Read the model definition and answer for the solid it produces. Units are mm, in the model's axes. A direction names the side the tool comes from. Coordinates: 2 decimals unless noted, no trailing zeros. Loops run counter-clockwise (first coordinate to the right, second up) from the corner with the lowest first, then second, coordinate; pieces in that order, holes last. Notation, with made-up numbers: (-6.75, 63) -> (11.25, 63) arc R13 ccw to (11.25, 69) -> close; hole circle Ø6 at (-26, -1.75). An arc over 180 degrees is marked (long way). Answer in a Markdown table with one row per item.
```python
from build123d import *

# Parameters (mm, degrees)
BASE_EXTRUSION_DEPTH    = 5.04
ESQUISSE3_R             = 2.5
ENL_V_MAT_EXTRU_1_DEPTH = 8.920538702
ESQUISSE5_R             = 2.5
ESQUISSE5_R_2           = 2
BOSS_EXTRU_1_DEPTH      = 5.04


with BuildPart() as part:
    # Esquisse1 → Base-Extrusion (new body)
    with BuildSketch(Plane.XY):
        Polygon((4, -2.309401077), (4, 2.309401077), (0, 4.618802154), (-4, 2.309401077), (-4, -2.309401077), (0, -4.618802154), align=None)
    extrude(amount=-BASE_EXTRUSION_DEPTH)

    # Esquisse2 → Enlèvement de matière-Révolution1 (revolve, cut)
    with BuildSketch(Plane(origin=(0, 0, 0), x_dir=(1, 0, 0), z_dir=(0, 1, 0))):
        Polygon((-4, 0), (-9.364768035, 0), (-9.364768035, 5.04), (-4, 5.04), (-8.364768035, 2.52), align=None)
    revolve(axis=Axis((0, 0, -5.04), (0, 0, 1)), mode=Mode.SUBTRACT)

    # Esquisse3 → Enlèv. mat.-Extru.1 (cut, through all)
    with BuildSketch(Plane.XY):
        Circle(ESQUISSE3_R)
    extrude(amount=-ENL_V_MAT_EXTRU_1_DEPTH, mode=Mode.SUBTRACT)

    # Esquisse4 → Boss.-Révol.1 (revolve)
    with BuildSketch(Plane(origin=(0, 0, 0), x_dir=(0, 0, -1), z_dir=(1, 0, 0)), mode=Mode.PRIVATE) as boss_r_vol_1_sk:
        with BuildLine():
            Line((5.04, 4), (5.67, 4))
            ThreePointArc((5.67, 4), (6.115477272, 3.815477272), (6.3, 3.37))
            Line((6.3, 3.37), (6.3, 3.154700538))
            Line((6.3, 3.154700538), (5.775, 3.154700538))
            Line((5.775, 3.154700538), (5.775, 2.309401077))
            Line((5.775, 2.309401077), (5.04, 2.309401077))
            Line((5.04, 2.309401077), (5.04, 4))
        make_face()
    revolve(boss_r_vol_1_sk.sketch.rotate(Axis((0, 0, 0), (0, 0, -1)), 90), axis=Axis((0, 0, 0), (0, 0, -1)))

    # Esquisse5 → Boss.-Extru.1 (add)
    with BuildSketch(Plane.XY):
        Circle(ESQUISSE5_R)
        Circle(ESQUISSE5_R_2, mode=Mode.SUBTRACT)
    extrude(amount=-BOSS_EXTRU_1_DEPTH)


solid = part.part
```
1. A cutting plane is placed at A-A on z = -1.5. Give the vertices of the cut face in (x, y).
A:
| item | result |
|---|---|
| outline | (-4, -2.31) -> (0, -4.62) -> (4, -2.31) -> (4, 2.31) -> (0, 4.62) -> (-4, 2.31) -> close; hole circle Ø4 at (0, 0) |
2. The mould has two halves that part along Y. Classify faces 1 (the cylindrical face through (-0.867, 3.905, -5.359)), 2 (the cylindrical face through (0, -2, -2)), 3 (the conical face through (3.6, 2.07, -4.95)), 4 (the cylindrical face through (1.456, 2.799, -6.034)): pulls with the +Y half, pulls with the -Y half, needs draft (parallel to the pull), parting line crosses it, or undercut.
A:
| item | result |
|---|---|
| face 1 | parting line crosses it |
| face 2 | undercut |
| face 3 | pulls with the +Y half |
| face 4 | undercut |
3. A cutting plane is placed at B-B on z = -5.5. Give the vertices of the cut face in (x, y).
A:
| item | result |
|---|---|
| outline | circle Ø8 at (0, 0); hole circle Ø4.62 at (0, 0) |
4. A tool of negligible diameter and unlimited length cuts with its end or side. For faces 5 (the cylindrical face through (1.066, 2.049, -5.402)), 6 (the flat face through (2.028, 3.448, -2.485)), from which of +Z, -Z, +X, -X, +Y, -Y can it reach the whole face along a straight path? Write none if from no direction.
A:
| item | result |
|---|---|
| face 5 | -Z |
| face 6 | +Z, -Z, +X, +Y |
5. Find the intervals of material crossed by probe 1 along Z at (x, y) = (-2.5, 0) (3 decimals); probe 2 along Y at (x, z) = (0, -5.55); probe 3 along X at (y, z) = (-0.25, -5), in increasing order.
A:
| item | result |
|---|---|
| probe 1 | z = -5.775 to 0 |
| probe 2 | y = -4 to -2.31, 2.31 to 4 |
| probe 3 | x = -4 to -1.98, 1.98 to 4 |
6. Given pin 1 Ø2.5 at (x, y) = (-0.5, 1) entering from -Z (3 decimals); pin 2 Ø3 at (x, y) = (0, 0) entering from -Z (3 decimals); pin 3 Ø2 at (x, z) = (2, -5) entering from -Y, each flat-ended and moving along its own axis, determine where each tip first touches the part or whether it passes through.
A:
| item | result |
|---|---|
| pin 1 | stops at z = -5.775 |
| pin 2 | passes through |
| pin 3 | stops at y = -4.04 |
